Can you work these out from the model? Positions are in its coordinate system, mm. Face numbers are marked on the shaded views. Coordinates: 2 decimals unless noted, no trailing zeros. Loops run counter-clockwise (first coordinate to the right, second up) from the corner with the lowest first, then second, coordinate; pieces in that order, holes last. Notation, with made-up numbers: M 14.5,-31.75 L 69.5,-31.75 A18 cw 69.5,-4.75 Z; hole C 60.25,40 d2. An arc over 180 degrees is marked long. Return JSON: item names as keys, results as strings. Group by question number.
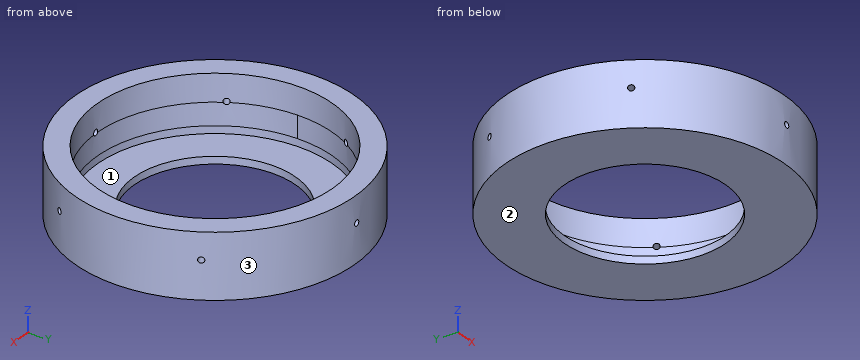
```python
from build123d import *
from build123d.topology import SkipClean

# Parameters (mm, degrees)
SKETCH_1_R               = 95
SKETCH_1_R_2             = 55
EXTRUDE_1_DEPTH          = 5
SKETCH_2_R               = 95
SKETCH_2_R_2             = 80
EXTRUDE_2_DEPTH          = 38.5
SKETCH_3_R               = 2
CUT_EXTRUDE_2_DEPTH      = 100
PATTERN_CIRCULAR_2_COUNT = 6
SKETCH_5_R               = 80
CUT_EXTRUDE_3_DEPTH      = 20
EXTRUDE_START            = 5
SKETCH_6_R               = 95
SKETCH_6_R_2             = 55
EXTRUDE_3_DEPTH          = 5


with BuildPart() as part:
    # Sketch 1 → Extrude 1 (new body)
    with BuildSketch(Plane.XY):
        Circle(SKETCH_1_R)
        Circle(SKETCH_1_R_2, mode=Mode.SUBTRACT)
    extrude(amount=EXTRUDE_1_DEPTH)

    # Sketch 2 → Extrude 2 (add)
    with BuildSketch(Plane.XY):
        Circle(SKETCH_2_R)
        Circle(SKETCH_2_R_2, mode=Mode.SUBTRACT)
    extrude(amount=EXTRUDE_2_DEPTH)

    # Sketch 3 → Cut-Extrude 2 (cut)
    with BuildSketch(Plane(origin=(0, 0, 0), x_dir=(1, 0, 0), z_dir=(0, 1, 0))):
        with Locations(Location((0, -20.6, 0), (0, 0, 270))):
            Circle(SKETCH_3_R)
    cut_extrude_2 = extrude(amount=-CUT_EXTRUDE_2_DEPTH, mode=Mode.SUBTRACT)

    # Pattern Circular 2: Cut-Extrude 2 ×6 about axis
    pattern_circular_2_axis = Axis((0, 0, 5), (0, 0, -1))
    for i in range(1, PATTERN_CIRCULAR_2_COUNT):
        add(cut_extrude_2.rotate(pattern_circular_2_axis, i * 360 / PATTERN_CIRCULAR_2_COUNT), mode=Mode.SUBTRACT)

    # Sketch 5 → Cut-Extrude 3 (cut)
    with SkipClean():  # the faces are left unmerged after this step: merging them gives an invalid solid
        with BuildSketch(Plane(origin=(0, 0, 0), x_dir=(-1, 0, 0), z_dir=(0, 0, -1))):
            Circle(SKETCH_5_R)
        extrude(amount=-CUT_EXTRUDE_3_DEPTH, mode=Mode.SUBTRACT)
    add(part.part.scale(1), mode=Mode.REPLACE)  # the faces are merged on a copy

    # Sketch 6 → Extrude 3 (add)
    with SkipClean():  # the faces are left unmerged after this step: merging them gives an invalid solid
        with BuildSketch(Plane(origin=(0, 0, 0), x_dir=(-1, 0, 0), z_dir=(0, 0, -1)).offset(EXTRUDE_START)):
            Circle(SKETCH_6_R)
            Circle(SKETCH_6_R_2, mode=Mode.SUBTRACT)
        extrude(amount=-EXTRUDE_3_DEPTH)


solid = part.part
```
1) Suppose I cut it at B-B, the plane z = 33.5. List the corners of the cut face in (x, y) for me, then the cut area to 3 significant figures.
2) Suppose I cut it at D-D, the plane x = -72.5. Give the number of separate pieces and of enclosed holes in the cut face, then the cut area to 3 significant figures.
3) If we mould it in two halves opening along X, with no side actions, what happens to the marked faces 1, 2 and 3? For each: +X half, -X half, draft (parallel to the pull), parting line (faces both ways), or undercut.
4) If I drill on line 1 (Y direction, x = 0, z = -2); line 2 (Z direction, x = 0, y = -88); line 3 (Y direction, x = 0, z = 26.75), over which ranges is the centre line in solid material (lowest first)? Write a range as from..to.
5) Suppose I cut it at C-C, the plane x = 7. List the corners of the cut face in (y, z) for me, then the cut area to 3 significant figures.
6) Suppose I cut it at A-A, the plane x = -32. List the corners of the cut face in (y, z) for me.
7) For pin 1 (2 mm diameter, centred on x = -8, z = 26, fed in from -Y); pin 2 (3 mm diameter, centred on y = -55, z = 5.5, fed in from +X); pin 3 (1 mm diameter, centred on x = 27, z = 18.5, fed in from +Y); pin 4 (8 mm diameter, centred on x = -60.5, y = 75, fed in from -Z), each with a flat end and sliding along its axis, tell me the tip position at first contact or that it passes through.
Returned:
{
 "1": {"outline": "C 0,0 d190; hole C 0,0 d160", "area": "8,250 mm²"},
 "2": {"separate pieces": "1", "enclosed holes": "2", "area": "2,710 mm²"},
 "3": {"face 1": "undercut", "face 2": "draft", "face 3": "parting line"},
 "4": {"line 1": "y = -95..-55, 55..95", "line 2": "z = -5..18.6, 22.6..38.5", "line 3": "y = -95..-80, 80..95"},
 "5": {"outline": "M -94.74,-5 L -54.55,-5 L -54.55,0 L -79.69,0 L -79.69,38.5 L -94.74,38.5 Z; M 54.55,-5 L 94.74,-5 L 94.74,38.5 L 79.69,38.5 L 79.69,0 L 54.55,0 Z", "area": "1,560 mm²"},
 "6": {"outline": "M -89.45,-5 L -44.73,-5 L -44.73,0 L -73.32,0 L -73.32,38.5 L -89.45,38.5 Z; M 44.73,-5 L 89.45,-5 L 89.45,38.5 L 73.32,38.5 L 73.32,0 L 44.73,0 Z"},
 "7": {"pin 1": "stops at y = -94.74", "pin 2": "stops at x = 78.5", "pin 3": "stops at y = 91.23", "pin 4": "stops at z = -5"}
}
